Design review of the part built by this model. Coordinates are the model's own, in mm. A direction names the side the tool comes from. Give positions to 0.01 mm unless a question says otherwise; leave off trailing zeros. Loops run counter-clockwise (first coordinate to the right, second up) from the corner with the lowest first, then second, coordinate; pieces in that order, holes last. Notation, with made-up numbers: M 58,89.5 L 78,89.5 A28 cw 78,122.5 Z; hole C 74.5,58 d8. An arc over 180 degrees is marked long. Use a Markdown table: item, result. Add a question column.
(1) Draft analysis for pull direction X (two halves, no side actions). For faces 1 (the face through (-15, -5, 2)), 2 (the face through (6.466, 2.681, 10.423)), 3 (the face through (0, 0, 5)), state which applies: pulls with the +X half, pulls with the -X half, needs draft (parallel to the pull), parting line crosses it, or undercut.
(2) Add section C-C, the plane z = 12. Give the boundary of the cut face in (x, y), then the cut area to 3 significant figures.
(3) Add section D-D, the plane y = -5.25. Give the boundary of the cut face in (x, z).
(4) Insertion check: pin 1 Ø5.5 at (x, y) = (0, 0) entering from +Z. The pin has a flat end and moves straight along its axis. Give the tip position at first contact, or say it passes through.
(5) Add section B-B, the plane z = 3.5. Give the boundary of the cut face in (x, y), then the cut area to 3 significant figures.
(6) For faces 4 (the face through (-0.59, -4.46, 10.42)), 5 (the face through (13, 3, 2)), 6 (the face through (-13, 3, 2)), list the 3-axis set-ups (+Z, -Z, +X, -X, +Y, -Y) from which the entire face can be reached by the end or side of a thin tool; tool diameter is ignored.
(7) For probe 1 along Y at (x, z) = (0, 11); probe 2 along Z at (x, y) = (1.5, 3.75); probe 3 along Y at (x, z) = (-9.25, 3), list the stretches that pass through material, from the lowest coordinate up.
(8) Add section A-A, the plane x = 0. Give the boundary of the cut face in (y, z).
Autodesk Inventor part; units mm, degrees
ref_plane "YZ Plane" through (0, 0, 0) normal (1, 0, 0) x (0, 1, 0)
ref_plane "XZ Plane" through (0, 0, 0) normal (0, 1, 0) x (-1, 0, 0)
ref_plane "XY Plane" through (0, 0, 0) normal (0, 0, 1) x (1, 0, 0)
sketch "草图1" plane through (0, 0, 0) normal (0, 0, 1) x (1, 0, 0)
  line L0 (-15, 7.5) -> (15, 7.5)
  line L1 (15, -7.5) -> (-15, -7.5)
  line L2 (-15, 7.5) -> (15, -7.5) construction
  line L3 (15, 7.5) -> (-15, -7.5) construction
  arc A0 (11, 3) -> (11, -3) centre (11, 0) ccw
  arc A1 (-11, -3) -> (-11, 3) centre (-11, 0) ccw
  line L4 (-11, 3) -> (-15, 3)
  line L5 (-11, -3) -> (-15, -3)
  line L6 (11, 3) -> (15, 3)
  line L7 (11, -3) -> (15, -3)
  line L8 (-15, -7.5) -> (-15, -3)
  line L9 (-15, 3) -> (-15, 7.5)
  line L10 (15, 7.5) -> (15, 3)
  line L11 (15, -3) -> (15, -7.5)
  point P0 (0, 0)
  dimension "d0" = 30
  dimension "d1" = 15
  dimension "d4" = 6
  dimension "d5" = 6
  dimension "d6" = 22
  dimension "d7" = 63.435
  dimension "d8" = 63.435
  dimension "d9" = 4.5
  dimension "d10" = 4
  dimension "d11" = 4
extrude "拉伸1" add sketch "草图1" along normal blind 5
sketch "草图2" plane through (0, 0, 5) normal (0, 0, 1) x (1, 0, 0)
  circle A0 centre (0, 0) radius 4.5
  circle A1 centre (0, 0) radius 7
  dimension "d14" = 9
  dimension "d15" = 14
extrude "拉伸2" add sketch "草图2" along normal blind 11
properties part number "2-3"
Established:
| question | item | result |
|---|---|---|
| 1 | face 1 | pulls with the -X half |
| 1 | face 2 | parting line crosses it |
| 1 | face 3 | undercut |
| 2 | outline | C 0,0 d14; hole C 0,0 d9 |
| 2 | area | 90.3 mm^2 |
| 3 | outline | M -15,0 L 15,0 L 15,5 L 4.63,5 L 4.63,16 L -4.63,16 L -4.63,5 L -15,5 Z |
| 4 | pin 1 | z = 5 |
| 5 | outline | M -15,-7.5 L 15,-7.5 L 15,-3 L 11,-3 A3 cw 11,3 L 15,3 L 15,7.5 L -15,7.5 L -15,3 L -11,3 A3 cw -11,-3 L -15,-3 Z |
| 5 | area | 374 mm^2 |
| 6 | face 4 | +Z |
| 6 | face 5 | +Z, -Z, +X |
| 6 | face 6 | +Z, -Z, -X |
| 7 | probe 1 | -7 to -4.5, 4.5 to 7 |
| 7 | probe 2 | 0 to 5 |
| 7 | probe 3 | -7.5 to -2.44, 2.44 to 7.5 |
| 8 | outline | M -7.5,0 L 7.5,0 L 7.5,5 L 7,5 L 7,16 L 4.5,16 L 4.5,5 L -4.5,5 L -4.5,16 L -7,16 L -7,5 L -7.5,5 Z |
